```python
from build123d import *

# Parameters (mm, degrees)
SKETCH1_R           = 2.8
BOSS_EXTRUDE1_DEPTH = 45


with BuildPart() as part:
    # Sketch1 → Boss-Extrude1 (new body)
    with BuildSketch(Plane(origin=(0, 0, 0), x_dir=(1, 0, 0), z_dir=(0, 1, 0))):
        with BuildLine():
            Line((20, -3.55), (20, 4.65))
            Line((20, 4.65), (29, 4.65))
            ThreePointArc((29, 4.65), (29.707106781, 4.942893219), (30, 5.65))
            Line((30, 5.65), (30, 15.05))
            ThreePointArc((30, 15.05), (29.707106781, 15.757106781), (29, 16.05))
            Line((29, 16.05), (20, 16.05))
            Line((20, 16.05), (-20, 16.05))
            Line((-20, 16.05), (-29, 16.05))
            ThreePointArc((-29, 16.05), (-29.707106781, 15.757106781), (-30, 15.05))
            Line((-30, 15.05), (-30, 5.65))
            ThreePointArc((-30, 5.65), (-29.707106781, 4.942893219), (-29, 4.65))
            Line((-29, 4.65), (-20, 4.65))
            Line((-20, 4.65), (-20, -3.55))
            Line((-20, -3.55), (-29, -3.55))
            ThreePointArc((-29, -3.55), (-29.707106781, -3.842893219), (-30, -4.55))
            Line((-30, -4.55), (-30, -13.95))
            ThreePointArc((-30, -13.95), (-29.707106781, -14.657106781), (-29, -14.95))
            Line((-29, -14.95), (-20, -14.95))
            Line((-20, -14.95), (20, -14.95))
            Line((20, -14.95), (29, -14.95))
            ThreePointArc((29, -14.95), (29.707106781, -14.657106781), (30, -13.95))
            Line((30, -13.95), (30, -4.55))
            ThreePointArc((30, -4.55), (29.707106781, -3.842893219), (29, -3.55))
            Line((29, -3.55), (20, -3.55))
        make_face()
        with Locations(Location((0, 0, 0), (0, 0, 90))):
            Circle(SKETCH1_R, mode=Mode.SUBTRACT)
    extrude(amount=BOSS_EXTRUDE1_DEPTH)


solid = part.part
```
Model file for the job. Use its own axes, mm. A direction names the side the tool comes from. Give positions to 0.01 mm unless a question says otherwise; leave off trailing zeros. Loops run counter-clockwise (first coordinate to the right, second up) from the corner with the lowest first, then second, coordinate; pieces in that order, holes last. Notation, with made-up numbers: (68.25, -9.75) -> (114.25, -9.75) arc R31 cw to (114.25, 21.25) -> close; hole circle Ø4 at (49.25, -24.75). An arc over 180 degrees is marked (long way). Use CSV: the item, a comma, the result in double quotes. Start each with the question number.
1) Flat gauge pins, fed straight in: pin 1 Ø2.5 at (y, z) = (26.5, 1.5) entering from +X; pin 2 Ø6.5 at (y, z) = (15, -2) entering from -X. Where does each tip first touch, or does it go through?
2) Tool access for faces 4 (the flat face through (0, 22, -16.05)), 5 (the flat face through (-25, 22, -4.65)), 6 (the flat face through (20, 22, 0)): list every direction of +Z, -Z, +X, -X, +Y, -Y with a clear straight run to the whole face (end or side of a thin tool).
3) Slice it at A-A on x = 0. Give the cut face in (y, z), plus the area to 3 significant figures.
4) Wall check: line 1 (Z direction, x = 23, y = 32.5); line 2 (X direction, y = 33, z = 0); line 3 (Z direction, x = -2.5, y = 5). Give the ranges that are in metal, low to high.
5) Mould opens along X. For faces 1 (the flat face through (-24, 22, 3.55)), 2 (the flat face through (-30, 22, 9)), 3 (the cylindrical face through (-0.1, 22.2, 2.8)) say: released by +X, released by -X, zero draft, split by the parting line, or undercut.
6) Slice it at B-B on z = 0. Give the cut face in (x, y), plus the area to 3 significant figures.
7) Slice it at D-D on z = -4. Give the cut face in (x, y), plus the area to 3 significant figures.
8) Slice it at C-C on y = 37.5. Give the cut face in (x, z).
Computed values:
1,pin 1,"stops at x = 20"
1,pin 2,"stops at x = -29.92"
2,face 4,"-Z, +X, -X, +Y, -Y"
2,face 5,"-X, +Y, -Y"
2,face 6,"+X, +Y, -Y"
3,outline,"(0, -16.05) -> (45, -16.05) -> (45, -2.8) -> (0, -2.8) -> close; (0, 2.8) -> (45, 2.8) -> (45, 14.95) -> (0, 14.95) -> close"
3,area,"1,140 mm^2"
4,line 1,"z = -16.05 to -4.65, 3.55 to 14.95"
4,line 2,"x = -20 to -2.8, 2.8 to 20"
4,line 3,"z = -16.05 to -1.26, 1.26 to 14.95"
5,face 1,"zero draft"
5,face 2,"released by -X"
5,face 3,"undercut"
6,outline,"(-20, 0) -> (-2.8, 0) -> (-2.8, 45) -> (-20, 45) -> close; (2.8, 0) -> (20, 0) -> (20, 45) -> (2.8, 45) -> close"
6,area,"1,550 mm^2"
7,outline,"(-20, 0) -> (20, 0) -> (20, 45) -> (-20, 45) -> close"
7,area,"1,800 mm^2"
8,outline,"(-30, -15.05) arc R1 ccw to (-29, -16.05) -> (29, -16.05) arc R1 ccw to (30, -15.05) -> (30, -5.65) arc R1 ccw to (29, -4.65) -> (20, -4.65) -> (20, 3.55) -> (29, 3.55) arc R1 ccw to (30, 4.55) -> (30, 13.95) arc R1 ccw to (29, 14.95) -> (-29, 14.95) arc R1 ccw to (-30, 13.95) -> (-30, 4.55) arc R1 ccw to (-29, 3.55) -> (-20, 3.55) -> (-20, -4.65) -> (-29, -4.65) arc R1 ccw to (-30, -5.65) -> close; hole circle Ø5.6 at (0, 0)"
